Part model, mm, in its own coordinate system. A direction names the side the tool comes from. Give positions to 0.01 mm unless a question says otherwise; leave off trailing zeros. Write each loop counter-clockwise with the first axis right and the second up, starting at its lowest first coordinate (ties: lowest second). Pieces come first, ordered by that corner, then holes. Notation, with made-up numbers: M 87.25,-19.5 L 106.25,-19.5 A18 cw 106.25,-13.5 Z; hole C 23,-12 d9. An arc over 180 degrees is marked long. Answer as CSV lines item,"result". Start each with the question number.
Item 1: Band-saw the part on D-D, the plane z = -6. List the corners of the cut face in (x, y).
Item 2: Wall check: L1, parallel to Y at x = -1, z = 6.5; L2, parallel to X at y = 7, z = 3.75; L3, parallel to X at y = 18.5, z = 1.5. Give the ranges that are in metal, low to high. Write a range as from..to.
Item 3: Band-saw the part on B-B, the plane x = -3.5. List the corners of the cut face in (y, z), then the cut area to 3 significant figures.
Item 4: Band-saw the part on A-A, the plane z = 0. List the corners of the cut face in (x, y), then the cut area to 3 significant figures.
Item 5: Pin check, flat tips, straight feed: pin 1 (4 mm diameter, centred on x = -4, y = -9.5, fed in from -Z); pin 2 (1 mm diameter, centred on x = -3, y = 9.5, fed in from +Z); pin 3 (4 mm diameter, centred on x = -4.5, y = 0.5, fed in from -Z). Stop position of each tip, or through.
Item 6: Band-saw the part on C-C, the plane y = 12. List the corners of the cut face in (x, z), then the cut area to 3 significant figures.
Item 7: 3-axis set-ups, long thin cutter, end or side, ignore diameter. For faces 1 (the cylindrical face through (-3.78, -17.35, 2.9)), 2 (the flat face through (0, 14.16, 5)), 3 (the flat face through (3.131, 0.198, 5.525)): which of +Z, -Z, +X, -X, +Y, -Y reach the whole face in a straight line?
from build123d import *

# Parameters (mm, degrees)
BOSS_EXTRUDE1_DEPTH = 14.1605
SKETCH2_R           = 4.7625
BOSS_EXTRUDE2_DEPTH = 20.6375


with BuildPart() as part:
    # Sketch1 → Boss-Extrude1 (new body, symmetric)
    with BuildSketch(Plane(origin=(0, 0, 0), x_dir=(1, 0, 0), z_dir=(0, 1, 0))):
        Polygon((6.35, -3.666174209), (6.35, 3.666174209), (0, 7.332348419), (-6.35, 3.666174209), (-6.35, -3.666174209), (0, -7.332348419), align=None)
    extrude(amount=BOSS_EXTRUDE1_DEPTH, both=True)

    # Sketch2 → Boss-Extrude2 (add, symmetric)
    with BuildSketch(Plane(origin=(0, 0, 0), x_dir=(1, 0, 0), z_dir=(0, 1, 0))):
        Circle(SKETCH2_R)
    extrude(amount=BOSS_EXTRUDE2_DEPTH, both=True)


solid = part.part
Output:
1,outline,"M -2.31,-14.16 L 2.31,-14.16 L 2.31,14.16 L -2.31,14.16 Z"
2,L1,"-14.16..14.16"
2,L2,"-6.2..6.2"
2,L3,"-4.52..4.52"
3,outline,"M -20.64,-3.23 L -14.16,-3.23 L -14.16,-5.31 L 14.16,-5.31 L 14.16,-3.23 L 20.64,-3.23 L 20.64,3.23 L 14.16,3.23 L 14.16,5.31 L -14.16,5.31 L -14.16,3.23 L -20.64,3.23 Z"
3,area,"385 mm²"
4,outline,"M -6.35,-14.16 L -4.76,-14.16 L -4.76,-20.64 L 4.76,-20.64 L 4.76,-14.16 L 6.35,-14.16 L 6.35,14.16 L 4.76,14.16 L 4.76,20.64 L -4.76,20.64 L -4.76,14.16 L -6.35,14.16 Z"
4,area,"483 mm²"
5,pin 1,"z = -6.18"
5,pin 2,"z = 5.89"
5,pin 3,"z = -5.89"
6,outline,"M -6.35,-3.67 L 0,-7.33 L 6.35,-3.67 L 6.35,3.67 L 0,7.33 L -6.35,3.67 Z"
6,area,"140 mm²"
7,face 1,"-Y"
7,face 2,"+Y"
7,face 3,"+Z, +X, +Y, -Y"
